Model file for the job. Use its own axes, mm. A direction names the side the tool comes from. Coordinates: 2 decimals unless noted, no trailing zeros. Order: outer loops, then holes, each group sorted by start corner. A loop starts at its lowest first (then second) coordinate and runs counter-clockwise, first axis right, second up. Notation, with made-up numbers: M 82.25,-23 L 118.25,-23 A9 ccw 118.25,-13 Z; hole C 17.5,-29 d8. An arc over 180 degrees is marked long. Return JSON: item names as keys, results as strings.
```python
from build123d import *

# Parameters (mm, degrees)
SKETCH1_W           = 40
SKETCH1_H           = 170
BOSS_EXTRUDE1_DEPTH = 3
SKETCH2_W           = 5
SKETCH2_H           = 5
CUT_EXTRUDE1_DEPTH  = 10


with BuildPart() as part:
    # Sketch1 → Boss-Extrude1 (new body)
    with BuildSketch(Plane(origin=(0, 0, 0), x_dir=(1, 0, 0), z_dir=(0, 1, 0))):
        with Locations((20, 85)):
            Rectangle(SKETCH1_W, SKETCH1_H)
    extrude(amount=BOSS_EXTRUDE1_DEPTH)

    # Sketch2 → Cut-Extrude1 (cut)
    with BuildSketch(Plane(origin=(0, 0, 0), x_dir=(1, 0, 0), z_dir=(0, 1, 0))):
        with Locations((2.5, 152.5)):
            Rectangle(SKETCH2_W, SKETCH2_H)
        with Locations((37.5, 17.5)):
            Rectangle(SKETCH2_W, SKETCH2_H)
        with Locations((2.5, 17.5)):
            Rectangle(SKETCH2_W, SKETCH2_H)
        with Locations((37.5, 152.5)):
            Rectangle(SKETCH2_W, SKETCH2_H)
    extrude(amount=CUT_EXTRUDE1_DEPTH, mode=Mode.SUBTRACT)


solid = part.part
```
Item 1: Wall check: line 1 (Z direction, x = 37, y = 1.05). Give the ranges that are in metal, low to high.
Check result:
{"line 1": "z = -170 to -155, -150 to -20, -15 to 0"}
Item 2: Saw through at B-B (z = -17). Write the cut outline in (x, y).
Check result:
{"outline": "M 5,0 L 35,0 L 35,3 L 5,3 Z"}
Item 3: Saw through at A-A (x = 3). Write the cut outline in (y, z).
Check result:
{"outline": "M 0,-170 L 3,-170 L 3,-155 L 0,-155 Z; M 0,-150 L 3,-150 L 3,-20 L 0,-20 Z; M 0,-15 L 3,-15 L 3,0 L 0,0 Z"}
Item 4: Pull direction Z, two halves, no side cores. Call faces 4 (the flat face through (0, 1, -162)), 5 (the flat face through (20, 1, -170)), 6 (the flat face through (2, 1, -20)), 7 (the flat face through (20, 1, 0)): +Z half, -Z half, draft (parallel to the pull), parting line (faces both ways), or undercut.
Check result:
{"face 4": "draft", "face 5": "-Z half", "face 6": "undercut", "face 7": "+Z half"}
Item 5: Drop flat-ended pins along their axis: pin 1 Ø1.5 at (y, z) = (0.5, -18.5) entering from +X; pin 2 Ø1.5 at (y, z) = (2, -152) entering from -X. Give the stop position or say it passes through.
Check result:
{"pin 1": "stops at x = 35", "pin 2": "stops at x = 5"}
Item 6: 3-axis set-ups, long thin cutter, end or side, ignore diameter. For faces 1 (the flat face through (2, 1, -155)), 2 (the flat face through (35, 1, -152)), 3 (the flat face through (0, 1, -7)): which of +Z, -Z, +X, -X, +Y, -Y reach the whole face in a straight line?
Check result:
{"face 1": "-X, +Y, -Y", "face 2": "+X, +Y, -Y", "face 3": "+Z, -Z, -X, +Y, -Y"}
